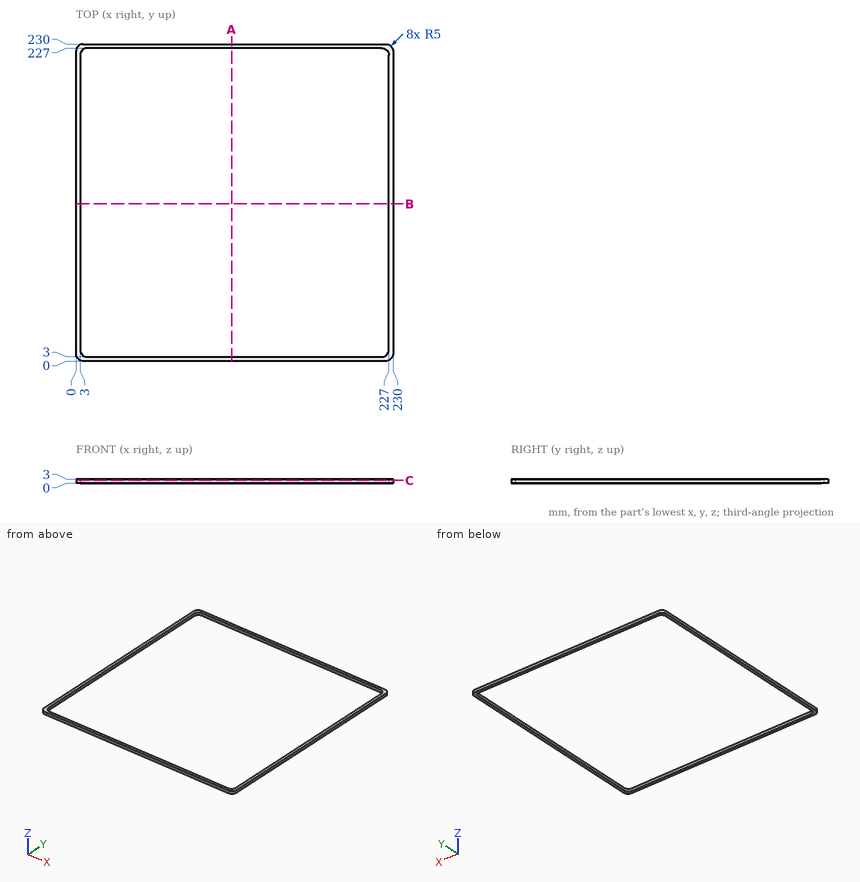
Source: three-view drawing plus pictorial views. Frame: mm from the lowest corner of the part. Round coordinates to 2 decimals unless told otherwise and drop trailing zeros. Loops run counter-clockwise (first coordinate to the right, second up) from the corner with the lowest first, then second, coordinate; pieces in that order, holes last.
Item 1: Line query: L1, parallel to Y at x = 99.5, z = 1.35. Output: solid intervals per line, ascending.
Checked values:
L1: y = 0 to 3, 227 to 230
Item 2: Section C-C, the plane z = 2. Output: boundary loops of the cut face in (x, y), plus the area to 3 significant figures.
Checked values:
outline: (0, 5) arc R5 ccw to (5, 0) - (225, 0) arc R5 ccw to (230, 5) - (230, 225) arc R5 ccw to (225, 230) - (5, 230) arc R5 ccw to (0, 225) - close; hole (3, 8) arc R5 ccw to (8, 3) - (222, 3) arc R5 ccw to (227, 8) - (227, 222) arc R5 ccw to (222, 227) - (8, 227) arc R5 ccw to (3, 222) - close
area: 2,720 mm2
Item 3: Section A-A, the plane x = 113. Output: boundary loops of the cut face in (y, z), plus the area to 3 significant figures.
Checked values:
outline: (0, 0) - (3, 0) - (3, 3) - (0, 3) - close; (227, 0) - (230, 0) - (230, 3) - (227, 3) - close
area: 18.0 mm2
